Here's how the part is built. I have some questions about the finished solid (model axes, mm). A direction names the side the tool comes from. Coordinates: 2 decimals unless noted, no trailing zeros. Order: outer loops, then holes, each group sorted by start corner. A loop starts at its lowest first (then second) coordinate and runs counter-clockwise, first axis right, second up. Notation, with made-up numbers: M -32,-10.5 L 24,-10.5 A20 cw 24,-0.5 Z; hole C 76,-20 d5. An arc over 180 degrees is marked long. One line per question, with ' | ' between items. Start each with the question number.
Autodesk Inventor part; units mm, degrees
ref_plane "YZ Plane" through (0, 0, 0) normal (1, 0, 0) x (0, 1, 0)
ref_plane "XZ Plane" through (0, 0, 0) normal (0, 1, 0) x (-1, 0, 0)
ref_plane "XY Plane" through (0, 0, 0) normal (0, 0, 1) x (1, 0, 0)
sketch "CONTOURS" plane through (0, 0, 0) normal (0, 0, 1) x (1, 0, 0)
  line L0 (2379.4087, 421.1241) -> (2379.4087, 437.5136)
  line L1 (2083.0497, 275.5979) -> (2083.0497, 256.5979)
  arc A0 (2075.0497, 256.5979) -> (2083.0497, 256.5979) centre (2079.0497, 256.5979) ccw
  line L2 (2075.0497, 256.5979) -> (2051.9087, 256.5979)
  line L3 (2051.9087, 256.5979) -> (2010.928, 256.5979)
  arc A1 (2003.428, 258.6076) -> (2010.928, 256.5979) centre (2010.928, 271.5979) ccw
  line L4 (2003.428, 258.6076) -> (1977.9087, 273.3411)
  arc A2 (1977.9087, 273.3411) -> (1971.9087, 269.877) centre (1975.9087, 269.877) ccw
  line L5 (1971.9087, 269.877) -> (1971.9087, 161.3189)
  arc A3 (1971.9087, 161.3189) -> (1977.9087, 157.8548) centre (1975.9087, 161.3189) ccw
  line L6 (1977.9087, 157.8548) -> (2003.428, 172.5883)
  arc A4 (2010.928, 174.5979) -> (2003.428, 172.5883) centre (2010.928, 159.5979) ccw
  line L7 (2010.928, 174.5979) -> (2051.9087, 174.5979)
  line L8 (2051.9087, 174.5979) -> (2075.0497, 174.5979)
  arc A5 (2083.0497, 174.5979) -> (2075.0497, 174.5979) centre (2079.0497, 174.5979) ccw
  line L9 (2083.0497, 174.5979) -> (2083.0497, 155.5979)
  arc A6 (2075.0497, 155.5979) -> (2083.0497, 155.5979) centre (2079.0497, 155.5979) ccw
  line L10 (2075.0497, 155.5979) -> (2053.0497, 155.5979)
  line L11 (2053.0497, 155.5979) -> (2053.0497, 46.9498)
  arc A7 (2053.0497, 46.9498) -> (2341.9087, 177.362) centre (1668.415, 1284.0168) ccw
  line L12 (2341.9087, 177.362) -> (2341.9087, 234.1241)
  arc A8 (2349.9087, 234.1241) -> (2341.9087, 234.1241) centre (2345.9087, 234.1241) ccw
  line L13 (2349.9087, 234.1241) -> (2409.4087, 234.1241)
  line L14 (2409.4087, 234.1241) -> (2409.4087, 275.172)
  arc A9 (2409.4087, 283.172) -> (2409.4087, 275.172) centre (2409.4087, 279.172) ccw
  line L15 (2409.4087, 283.172) -> (2425.9087, 283.172)
  line L16 (2425.9087, 283.172) -> (2425.9087, 301.172)
  line L17 (2425.9087, 301.172) -> (2417.4087, 301.172)
  arc A10 (2409.4087, 301.172) -> (2417.4087, 301.172) centre (2413.4087, 301.172) ccw
  line L18 (2409.4087, 301.172) -> (2409.4087, 421.1241)
  line L19 (2409.4087, 421.1241) -> (2387.4087, 421.1241)
  arc A11 (2379.4087, 421.1241) -> (2387.4087, 421.1241) centre (2383.4087, 421.1241) ccw
  line L20 (2379.4087, 437.5136) -> (2379.1671, 437.3833)
  line L21 (2379.1671, 437.3833) -> (2378.928, 437.2484)
  line L22 (2378.928, 437.2484) -> (2353.7677, 422.7221)
  arc A12 (2346.2677, 427.0523) -> (2353.7677, 422.7221) centre (2351.2677, 427.0523) ccw
  line L23 (2346.2677, 427.0523) -> (2346.2677, 622.1959)
  arc A13 (2353.7677, 626.526) -> (2346.2677, 622.1959) centre (2351.2677, 622.1959) ccw
  line L24 (2353.7677, 626.526) -> (2378.928, 611.9997)
  line L25 (2378.928, 611.9997) -> (2379.1671, 611.8648)
  line L26 (2379.1671, 611.8648) -> (2379.4087, 611.7346)
  line L27 (2379.4087, 611.7346) -> (2379.4087, 628.1241)
  arc A14 (2387.4087, 628.1241) -> (2379.4087, 628.1241) centre (2383.4087, 628.1241) ccw
  line L28 (2387.4087, 628.1241) -> (2409.4087, 628.1241)
  line L29 (2409.4087, 628.1241) -> (2409.4087, 748.0761)
  arc A15 (2417.4087, 748.0761) -> (2409.4087, 748.0761) centre (2413.4087, 748.0761) ccw
  line L30 (2417.4087, 748.0761) -> (2425.9087, 748.0761)
  line L31 (2425.9087, 748.0761) -> (2425.9087, 766.0761)
  line L32 (2425.9087, 766.0761) -> (2409.4087, 766.0761)
  arc A16 (2409.4087, 774.0761) -> (2409.4087, 766.0761) centre (2409.4087, 770.0761) ccw
  line L33 (2409.4087, 774.0761) -> (2409.4087, 786.8861)
  arc A17 (2409.4087, 786.8861) -> (2401.6988, 788.3816) centre (2405.4087, 786.8861) ccw
  arc A18 (2066.9087, 401.2195) -> (2401.6988, 788.3816) centre (1668.7587, 1083.8435) ccw
  line L34 (2066.9087, 401.2195) -> (2066.9087, 392.5981)
  arc A19 (2066.9087, 384.5981) -> (2066.9087, 392.5981) centre (2066.9087, 388.5981) ccw
  line L35 (2066.9087, 384.5981) -> (2053.0497, 384.5981)
  line L36 (2053.0497, 384.5981) -> (2053.0497, 275.5979)
  line L37 (2053.0497, 275.5979) -> (2075.0497, 275.5979)
  arc A20 (2083.0497, 275.5979) -> (2075.0497, 275.5979) centre (2079.0497, 275.5979) ccw
sketch "HOLES" plane through (0, 0, 0) normal (0, 0, 1) x (1, 0, 0)
  arc A0 (2359.9087, 385.1025) -> (2355.9087, 381.1025) centre (2359.9087, 381.1025) ccw
  line L0 (2359.9087, 385.1025) -> (2389.9087, 385.1025)
  arc A1 (2393.9087, 381.1025) -> (2389.9087, 385.1025) centre (2389.9087, 381.1025) ccw
  line L1 (2393.9087, 381.1025) -> (2393.9087, 370.1025)
  arc A2 (2389.9087, 366.1025) -> (2393.9087, 370.1025) centre (2389.9087, 370.1025) ccw
  line L2 (2389.9087, 366.1025) -> (2359.9087, 366.1025)
  arc A3 (2355.9087, 370.1025) -> (2359.9087, 366.1025) centre (2359.9087, 370.1025) ccw
  line L3 (2355.9087, 370.1025) -> (2355.9087, 381.1025)
sketch "LETTERS" plane through (0, 0, 0) normal (0, 0, 1) x (1, 0, 0)
  arc A0 (2211.6565, 303.9645) -> (2200.9951, 304.2164) centre (2206.3294, 304.2452) ccw
  line L0 (2200.9964, 295.3379) -> (2200.9964, 303.7395)
  arc A1 (2200.9964, 303.7395) -> (2191.9817, 303.7395) centre (2196.489, 303.7395) ccw
  line L1 (2191.9817, 303.7395) -> (2191.9817, 295.3379)
  line L2 (2211.6565, 295.3379) -> (2211.6565, 299.2505)
  line L3 (2211.6565, 299.2505) -> (2211.6639, 304.2373)
  line L4 (2191.9817, 295.3379) -> (2211.6565, 295.3379)
extrude "Extrusion3" add sketch "CONTOURS" along normal blind 18
properties part number "Support B" material "Wood (Birch)"
1. I need wall thicknesses on line 1 (X direction, y = 183, z = 8); line 2 (X direction, y = 373, z = 12.25); line 3 (Y direction, x = 2057, z = 12.5). Which ranges of each line are inside material? Lowest first, please.
2. Imagine slicing it at B-B (x = 2097). List the corners of the cut face in (y, z) for me, then the cut area to 3 significant figures.
3. Which directions (+Z, -Z, +X, -X, +Y, -Y) give clear straight access to the entire face, cutting with the end or side of a thin tool? Please do faces 1 (the face through (2418, 283.172, 9)), 2 (the face through (2083.05, 165, 9)), 3 (the face through (2399, 421.124, 9)).
4. We'd pull the mould along Y, two halves only. Please class faces 4 (the face through (2409.409, 254, 9)), 5 (the face through (2379.409, 429, 9)), 6 (the face through (2203.5, 104.2, 8.9)): released by +Y, released by -Y, zero draft, split by the parting line, or undercut.
5. Imagine slicing it at A-A (y = 320). List the corners of the cut face in (x, z) for me.
6. Will these pins go through, and if not, where does the flat tip stop? pin 1 (2.5 mm diameter, centred on y = 398, z = 9.5, fed in from -X); pin 2 (5.5 mm diameter, centred on x = 2068.5, z = 12, fed in from -Y); pin 3 (6.5 mm diameter, centred on y = 783.5, z = 8, fed in from +X); pin 4 (5 mm diameter, centred on x = 2045.5, y = 220.5, fed in from -Z).
Entries:
1) line 1: 1971.91 to 2341.91 | line 2: 2053.05 to 2409.41 | line 3: 48.18 to 155.6, 174.6 to 256.6, 275.6 to 384.6
2) outline: M 61.48,0 L 419.68,0 L 419.68,18 L 61.48,18 Z | area: 6,450 mm²
3) face 1: +Z, -Z, +X, -Y | face 2: +Z, -Z | face 3: +Z, -Z, +X
4) face 4: zero draft | face 5: undercut | face 6: released by -Y
5) outline: M 2053.05,0 L 2409.41,0 L 2409.41,18 L 2053.05,18 Z
6) pin 1: x = 2066.91 | pin 2: y = 50.97 | pin 3: x = 2409.41 | pin 4: z = 0
